Read the model definition and answer for the solid it produces. Units are mm, in the model's axes. Face numbers are marked on the shaded views. A direction names the side the tool comes from. Coordinates: 2 decimals unless noted, no trailing zeros. Order: outer loops, then holes, each group sorted by start corner. A loop starts at its lowest first (then second) coordinate and runs counter-clockwise, first axis right, second up. Notation, with made-up numbers: (-3.75, 43) - (37.25, 43) arc R26 cw to (37.25, 72) - close; hole circle Ø3 at (-6, 55.25). An arc over 180 degrees is marked (long way). Use one line per item in the form item = value. Start each with the question number.
from build123d import *

# Parameters (mm, degrees)
F0_R     = 10
F1_DEPTH = 30
F2_R     = 5
F3_R     = 5
F4_DEPTH = 10.001


with BuildPart() as f1:
    # F0 (on Front) → F1 (new body, symmetric)
    with BuildSketch(Plane.XZ):
        with BuildLine():
            ThreePointArc((24.494897, -10), (20.621914, -8.162278), (19.595918, -4))
            ThreePointArc((19.595918, -4), (0, 20), (-19.595918, -4))
            ThreePointArc((-19.595918, -4), (-20.621914, -8.162278), (-24.494897, -10))
            Line((-24.494897, -10), (-60, -10))
            Line((-60, -10), (-60, -20))
            Line((-60, -20), (60, -20))
            Line((60, -20), (60, -10))
            Line((60, -10), (24.494897, -10))
        make_face()
        Circle(F0_R, mode=Mode.SUBTRACT)
    extrude(amount=F1_DEPTH, both=True)

    # F2
    f2_edges = [f1.edges().sort_by_distance(p)[0] for p in [
        (60, 0, -10),
        (-60, 0, -10),
    ]]
    fillet(f2_edges, radius=F2_R)

    # F3 (on face) → F4 (cut, through all)
    with BuildSketch(Plane.XY.offset(-10)):
        with Locations((-40, 15)):
            Circle(F3_R)
        with Locations((-40, -15)):
            Circle(F3_R)
        with Locations((40, -15)):
            Circle(F3_R)
        with Locations((40, 15)):
            Circle(F3_R)
    extrude(amount=-F4_DEPTH, mode=Mode.SUBTRACT)


solid = f1.part
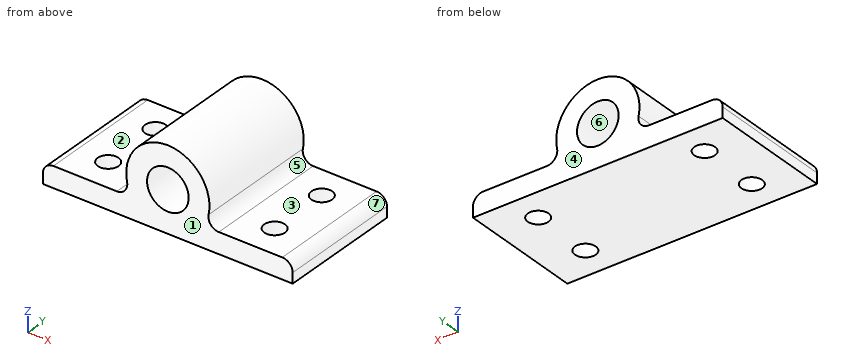
Q1. Which of the six approach directions +Z, -Z, +X, -X, +Y, -Y give full straight-line access (tool end or side, diameter ignored) to the marked faces 1, 2 and 3?
Q2. A cutting plane is placed at A-A (x = -40). Give the vertices of the cut face in (y, z), then the cut area to 3 significant figures.
Q3. A cutting plane is placed at C-C (y = -15). Give the vertices of the cut face in (x, z), then the cut area to 3 significant figures.
Q4. A cutting plane is placed at D-D (x = 0). Give the vertices of the cut face in (y, z).
Q5. For a pull along Z with two mould halves and no side action, classify the marked faces 4, 5, 6 and 7 as +Z half, -Z half, draft (parallel to the pull), parting line (faces both ways), or undercut.
Q6. A cutting plane is placed at B-B (z = 0). Give the vertices of the cut face in (x, y).
Q7. Consider probe 1 along Y at (x, z) = (-40, -16.75); probe 2 along Z at (x, y) = (0, 8); probe 3 along X at (y, z) = (13, -18). Determine where each line is inside the solid, lowest interval first.
Q8. Given P1, Ø4, axis at y = -13.5, z = -5.5, coming from the -X side; P2, Ø12, axis at y = 19.5, z = 4, coming from the +X side; P3, Ø2, axis at y = -23, z = 5.5, coming from the +X side, each flat-ended and moving along its own axis, determine where each tip first touches the part or whether it passes through.
Result sheet:
q1.face_1 = +Z, -Z, +X, -X, -Y
q1.face_2 = +Z, -X, +Y, -Y
q1.face_3 = +Z, +X, +Y, -Y
q2.outline = (-30, -20) - (-20, -20) - (-20, -10) - (-30, -10) - close; (-10, -20) - (10, -20) - (10, -10) - (-10, -10) - close; (20, -20) - (30, -20) - (30, -10) - (20, -10) - close
q2.area = 400 mm^2
q3.outline = (-60, -20) - (-45, -20) - (-45, -10) - (-55, -10) arc R5 ccw to (-60, -15) - close; (-35, -20) - (35, -20) - (35, -10) - (24.49, -10) arc R5 cw to (19.6, -4) arc R20 ccw (long way) to (-19.6, -4) arc R5 cw to (-24.49, -10) - (-35, -10) - close; (45, -20) - (60, -20) - (60, -15) arc R5 ccw to (55, -10) - (45, -10) - close; hole circle Ø20 at (0, 0)
q3.area = 1,710 mm^2
q4.outline = (-30, -20) - (30, -20) - (30, -10) - (-30, -10) - close; (-30, 10) - (30, 10) - (30, 20) - (-30, 20) - close
q5.face_4 = draft
q5.face_5 = undercut
q5.face_6 = undercut
q5.face_7 = +Z half
q6.outline = (-20, -30) - (-10, -30) - (-10, 30) - (-20, 30) - close; (10, -30) - (20, -30) - (20, 30) - (10, 30) - close
q7.probe_1 = -30 to -20, -10 to 10, 20 to 30
q7.probe_2 = -20 to -10, 10 to 20
q7.probe_3 = -60 to -44.58, -35.42 to 35.42, 44.58 to 60
q8.P1 = -20.16
q8.P2 = 20
q8.P3 = 19.49
